```python
from build123d import *

# Parameters (mm, degrees)
BOSS_EXTRU_1_DEPTH      = 8
BOSS_EXTRU_2_DEPTH      = 15
CONG_1_R                = 20
CONG_2_R                = 4
ESQUISSE3_R             = 7.5
BOSS_EXTRU_3_DEPTH      = 8
ENL_V_MAT_EXTRU_1_DEPTH = 172.56339936
ESQUISSE5_W             = 8
ESQUISSE5_H             = 15
ENL_V_MAT_EXTRU_2_DEPTH = 7.5
ESQUISSE6_W             = 8
ESQUISSE6_H             = 15
ENL_V_MAT_EXTRU_3_DEPTH = 32.5
ESQUISSE7_R             = 1.5
ENL_V_MAT_EXTRU_4_DEPTH = 8
D_GAGEMENT_M31_D        = 3.4
D_GAGEMENT_M31_DEPTH    = 10
D_GAGEMENT_M31_TIP      = 1.021463052
ESQUISSE10_R            = 1.5
ENL_V_MAT_EXTRU_5_DEPTH = 8
D_GAGEMENT_M32_D        = 3.4
D_GAGEMENT_M32_DEPTH    = 10
D_GAGEMENT_M32_TIP      = 1.021463052


with BuildPart() as part:
    # Esquisse1 → Boss.-Extru.1 (new body)
    with BuildSketch(Plane.XY):
        Polygon((64, 0), (64, 124.188364041), (0, 147.482459034), (2.736161147, 155), (68, 131.245905283), (133.263838853, 155), (136, 147.482459034), (72, 124.188364041), (72, 0), align=None)
    extrude(amount=BOSS_EXTRU_1_DEPTH)

    # Esquisse2 → Boss.-Extru.2 (add)
    with BuildSketch(Plane(origin=(0, 0, 0), x_dir=(-1, 0, 0), z_dir=(0, 0, -1))):
        Polygon((-132.241229517, 146.11437846), (-136, 147.482459034), (-133.263838853, 155), (-125.746297887, 152.263838853), (-127.11437846, 148.50506837), align=None)
        Polygon((0, 147.482459034), (-3.758770483, 146.11437846), (-8.88562154, 148.50506837), (-10.253702113, 152.263838853), (-2.736161147, 155), align=None)
    extrude(amount=BOSS_EXTRU_2_DEPTH)

    # Congé1
    cong_1_edges = [part.edges().sort_by_distance(p)[0] for p in [
        (64, 124.188364041, 4),
        (68, 131.245905283, 4),
        (72, 124.188364041, 4),
    ]]
    fillet(cong_1_edges, radius=CONG_1_R)

    # Congé2
    cong_2_edges = [part.edges().sort_by_distance(p)[0] for p in [
        (134.631919427, 151.241229517, 8),
        (1.368080573, 151.241229517, 8),
    ]]
    fillet(cong_2_edges, radius=CONG_2_R)

    # Esquisse3 → Boss.-Extru.3 (add)
    with BuildSketch(Plane.ZY.offset(-64)):
        with Locations((4, 0)):
            Circle(ESQUISSE3_R)
    extrude(amount=-BOSS_EXTRU_3_DEPTH)

    # Esquisse4 → Enlèv. mat.-Extru.1 (cut, through all)
    with BuildSketch(Plane.ZY.offset(-64)):
        with BuildLine():
            Line((2.25357508, 2.8), (5.74642492, 2.8))
            ThreePointArc((5.74642492, 2.8), (4, -3.3), (2.25357508, 2.8))
        make_face()
    extrude(amount=-ENL_V_MAT_EXTRU_1_DEPTH, mode=Mode.SUBTRACT)

    # Esquisse5 → Enlèv. mat.-Extru.2 (cut)
    with BuildSketch(Plane(origin=(0, 0, 0), x_dir=(1, 0, 0), z_dir=(0, 1, 0))):
        with Locations((68, -4)):
            Rectangle(ESQUISSE5_W, ESQUISSE5_H)
    extrude(amount=-ENL_V_MAT_EXTRU_2_DEPTH, mode=Mode.SUBTRACT)

    # Esquisse6 → Enlèv. mat.-Extru.3 (cut)
    with BuildSketch(Plane.XZ):
        with Locations((68, 4)):
            Rectangle(ESQUISSE6_W, ESQUISSE6_H)
    extrude(amount=-ENL_V_MAT_EXTRU_3_DEPTH, mode=Mode.SUBTRACT)

    # Esquisse7 → Enlèv. mat.-Extru.4 (cut)
    with BuildSketch(Plane.ZY.offset(-64)):
        with Locations(Location((4, 40.5, 0), (0, 0, 270))):
            Circle(ESQUISSE7_R)
    extrude(amount=-ENL_V_MAT_EXTRU_4_DEPTH, mode=Mode.SUBTRACT)

    # Dégagement M31
    with Locations(Plane.ZY.offset(-64)):
        with Locations((4, 40.5)):
            Hole(D_GAGEMENT_M31_D / 2, depth=D_GAGEMENT_M31_DEPTH)
            with Locations((0, 0, -(D_GAGEMENT_M31_DEPTH + D_GAGEMENT_M31_TIP / 2))):  # 118° drill point
                Cone(0, D_GAGEMENT_M31_D / 2, D_GAGEMENT_M31_TIP, mode=Mode.SUBTRACT)

    # Esquisse10 → Enlèv. mat.-Extru.5 (cut)
    with BuildSketch(Plane.XY.offset(8)):
        with Locations((68, 35.5)):
            Circle(ESQUISSE10_R)
        with Locations((68, 45.5)):
            Circle(ESQUISSE10_R)
    extrude(amount=-ENL_V_MAT_EXTRU_5_DEPTH, mode=Mode.SUBTRACT)

    # Dégagement M32
    with Locations(Plane(origin=(0, 0, 0), x_dir=(-1, 0, 0), z_dir=(0, 0, -1))):
        with Locations((-68, 45.5), (-68, 35.5)):
            Hole(D_GAGEMENT_M32_D / 2, depth=D_GAGEMENT_M32_DEPTH)
            with Locations((0, 0, -(D_GAGEMENT_M32_DEPTH + D_GAGEMENT_M32_TIP / 2))):  # 118° drill point
                Cone(0, D_GAGEMENT_M32_D / 2, D_GAGEMENT_M32_TIP, mode=Mode.SUBTRACT)


solid = part.part
```
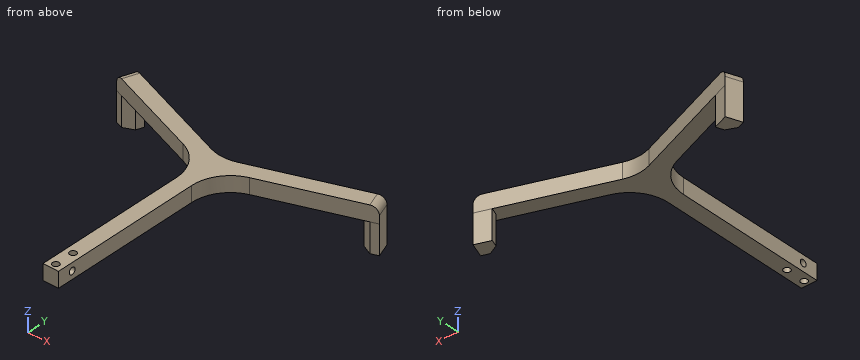
Geometry check sheet. Reference: the model listing, model coordinates, mm. Round coordinates to 2 decimals unless told otherwise and drop trailing zeros. Order: outer loops, then holes, each group sorted by start corner. A loop starts at its lowest first (then second) coordinate and runs counter-clockwise, first axis right, second up. Notation, with made-up numbers: (-4, 87.25) -> (38, 87.25) arc R20 ccw to (38, 94.25) -> close; hole circle Ø10 at (9.5, 29.25). An arc over 180 degrees is marked (long way). Return JSON: item names as keys, results as strings. Group by question number.
Q1. Section check C-C, the plane z = -8.75. Record the boundary of the cut face in (x, y), plus the area to 3 significant figures.
Q2. Material ranges on probe 1 along Y at (x, z) = (68, 2.25); probe 2 along Y at (x, z) = (68, 4); probe 3 along Y at (x, z) = (68, 3.25), recorded low to high. Write a range as from..to.
Q3. Gauge pin test, flat ends, axial feed: pin 1 (4.5 mm diameter, centred on y = 40.5, z = 4, fed in from -X); pin 2 (2 mm diameter, centred on x = 78, z = 1, fed in from -Y); pin 3 (10 mm diameter, centred on y = 53, z = -1.5, fed in from +X). Record the tip position at first contact, or that the pin passes through.
Q4. Section check B-B, the plane y = 45.5. Record the boundary of the cut face in (x, z).
Q5. Section check D-D, the plane x = 114.5. Record the boundary of the cut face in (y, z), plus the area to 3 significant figures.
Q6. Section check A-A, the plane x = 68. Record the boundary of the cut face in (y, z), plus the area to 3 significant figures.
Numbers:
{
 "1": {"outline": "(0, 147.48) -> (3.76, 146.11) -> (8.89, 148.51) -> (10.25, 152.26) -> (2.74, 155) -> close; (125.75, 152.26) -> (127.11, 148.51) -> (132.24, 146.11) -> (136, 147.48) -> (133.26, 155) -> close", "area": "112 mm^2"},
 "2": {"probe 1": "32.5..33.8, 37.2..43.8, 47.2..132.53", "probe 2": "32.5..33.8, 37.2..38.8, 42.2..43.8, 47.2..132.53", "probe 3": "32.5..33.8, 37.2..38.97, 42.03..43.8, 47.2..132.53"},
 "3": {"pin 1": "x = 64", "pin 2": "y = 123.41", "pin 3": "x = 72"},
 "4": {"outline": "(64, 0) -> (66.3, 0) -> (66.3, 8) -> (64, 8) -> close; (69.7, 0) -> (72, 0) -> (72, 8) -> (69.7, 8) -> close"},
 "5": {"outline": "(139.66, 0) -> (148.17, 0) -> (148.17, 8) -> (139.66, 8) -> close", "area": "68.1 mm^2"},
 "6": {"outline": "(32.5, 0) -> (33.8, 0) -> (33.8, 8) -> (32.5, 8) -> close; (37.2, 0) -> (43.8, 0) -> (43.8, 8) -> (37.2, 8) -> close; (47.2, 0) -> (132.53, 0) -> (132.53, 8) -> (47.2, 8) -> close; hole circle Ø3.4 at (40.5, 4)", "area": "737 mm^2"}
}
